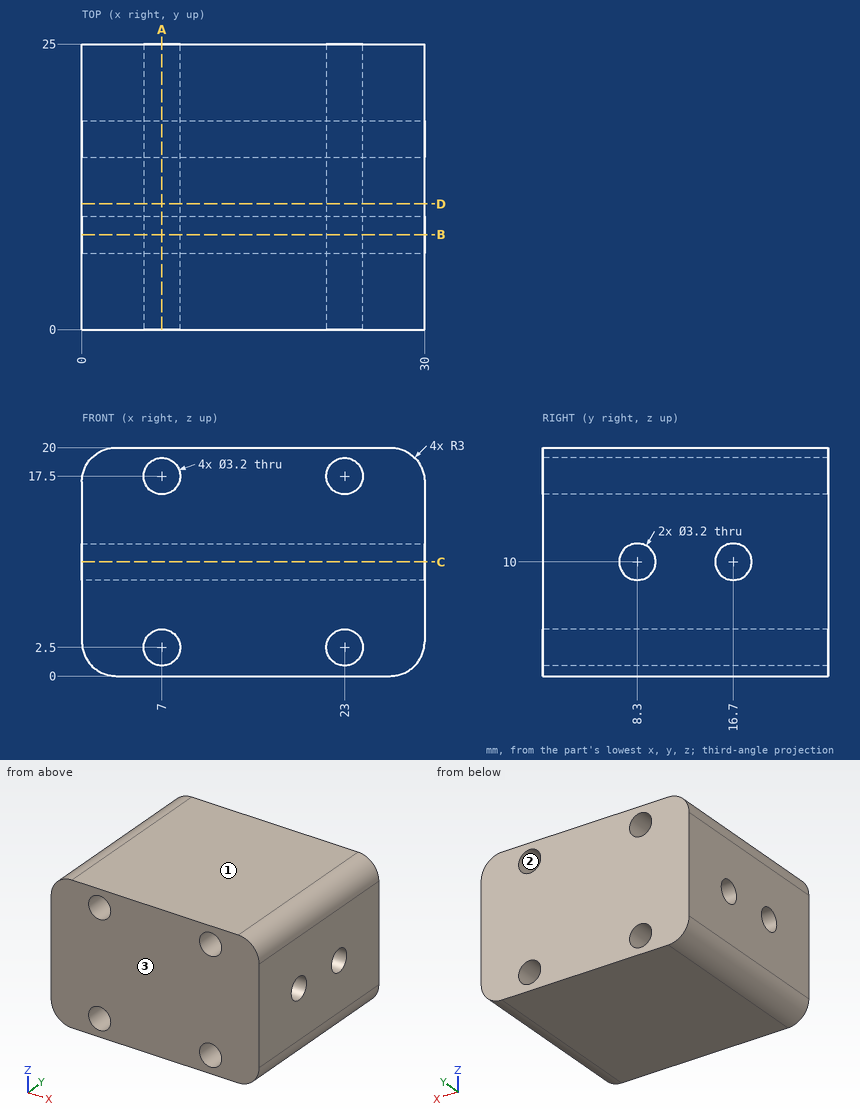
Verification items for this drawing (mm, ordinates from the low corner). Coordinates: 2 decimals unless noted, no trailing zeros. Write each loop counter-clockwise with the first axis right and the second up, starting at its lowest first coordinate (ties: lowest second). Pieces come first, ordered by that corner, then holes. Notation, with made-up numbers: M -8.5,68.25 L 30.5,68.25 A24 ccw 30.5,106.25 Z; hole C 27.25,13 d2. An arc over 180 degrees is marked long. Use CSV: the item, a comma, the result in double quotes.
Q1. Mould release check, pull along Z, two halves, no side actions. Record for the marked faces 1, 2 and 3: pulls with the +Z half, pulls with the -Z half, needs draft (parallel to the pull), parting line crosses it, or undercut.
Computed values:
face 1,"pulls with the +Z half"
face 2,"undercut"
face 3,"needs draft"
Q2. Section check B-B, the plane y = 8.3. Enter the section's corners in (x, z).
Computed values:
outline,"M 0,3 A3 ccw 3,0 L 27,0 A3 ccw 30,3 L 30,8.4 L 0,8.4 Z; M 0,11.6 L 30,11.6 L 30,17 A3 ccw 27,20 L 3,20 A3 ccw 0,17 Z; hole C 7,2.5 d3.2; hole C 7,17.5 d3.2; hole C 23,2.5 d3.2; hole C 23,17.5 d3.2"
Q3. Go/stop test with a flat-tipped pin: P1, Ø3, axis at x = 7, z = 2.5, coming from the +Y side. Record where the tip stops, or that it passes through.
Computed values:
P1,"through"
Q4. Section check C-C, the plane z = 10. Enter the section's corners in (x, y), and give its area (3 significant figures).
Computed values:
outline,"M 0,0 L 30,0 L 30,6.7 L 0,6.7 Z; M 0,9.9 L 30,9.9 L 30,15.1 L 0,15.1 Z; M 0,18.3 L 30,18.3 L 30,25 L 0,25 Z"
area,"558 mm²"
Q5. Section check D-D, the plane y = 11. Enter the section's corners in (x, z).
Computed values:
outline,"M 0,3 A3 ccw 3,0 L 27,0 A3 ccw 30,3 L 30,17 A3 ccw 27,20 L 3,20 A3 ccw 0,17 Z; hole C 7,2.5 d3.2; hole C 7,17.5 d3.2; hole C 23,2.5 d3.2; hole C 23,17.5 d3.2"
Q6. Thickness scan on line 1 along Z through (x, y) = (7, 10.25); line 2 along X through (y, z) = (24, 2.5); line 3 along X through (y, z) = (12.75, 2). Record the ranges inside material, lowest first. Write a range as [from, to].
Computed values:
line 1,"[0, 0.9], [4.1, 15.9], [19.1, 20]"
line 2,"[0.04, 5.4], [8.6, 21.4], [24.6, 29.96]"
line 3,"[0.17, 5.48], [8.52, 21.48], [24.52, 29.83]"
Q7. Section check A-A, the plane x = 7. Enter the section's corners in (y, z), and give its area (3 significant figures).
Computed values:
outline,"M 0,0 L 25,0 L 25,0.9 L 0,0.9 Z; M 0,4.1 L 25,4.1 L 25,15.9 L 0,15.9 Z; M 0,19.1 L 25,19.1 L 25,20 L 0,20 Z; hole C 8.3,10 d3.2; hole C 16.7,10 d3.2"
area,"324 mm²"
